```python
from build123d import *

# Parameters (mm, degrees)
SKETCH_1_W                         = 50
SKETCH_1_H                         = 140
SM_BASE_FLANGE_1_DEPTH             = 3
SM_EDGE_FLANGE_1_STRIP_W           = 13.4732
SM_EDGE_FLANGE_1_STRIP_H           = 3
SM_EDGE_FLANGE_1_STRIP_CUT_DEPTH   = 50
SM_EDGE_FLANGE_1_STRIP_2_W         = 13.4732
SM_EDGE_FLANGE_1_STRIP_2_H         = 3
SM_EDGE_FLANGE_1_STRIP_CUT_2_DEPTH = 50
SM_EDGE_FLANGE_1_DEPTH             = 50
SM_EDGE_FLANGE_1_BEND_DEPTH        = 50
SM_EDGE_FLANGE_2_STRIP_W           = 13.4732
SM_EDGE_FLANGE_2_STRIP_H           = 3
SM_EDGE_FLANGE_2_STRIP_CUT_DEPTH   = 50
SM_EDGE_FLANGE_2_STRIP_2_W         = 13.4732
SM_EDGE_FLANGE_2_STRIP_2_H         = 3
SM_EDGE_FLANGE_2_STRIP_CUT_2_DEPTH = 50
SM_EDGE_FLANGE_2_DEPTH             = 50
SM_EDGE_FLANGE_2_BEND_DEPTH        = 50
SKETCH_18_R                        = 6.5
CUT_EXTRUDE_1_DEPTH                = 179.686876966


# Sheet-metal steps are written as plain solids
with BuildPart() as part:
    # Sketch 1 → 基体-法兰1 (new body)
    with BuildSketch(Plane.XY):
        with Locations((25, 70)):
            Rectangle(SKETCH_1_W, SKETCH_1_H)
    extrude(amount=-SM_BASE_FLANGE_1_DEPTH)

    # 边线-法兰1 strip (across the edge) → 边线-法兰1 strip cut (cut)
    with BuildSketch(Plane(origin=(0, 140, -3), x_dir=(0, -1, 0), z_dir=(1, 0, 0))):
        with Locations((-6, -1.5)):
            Rectangle(SM_EDGE_FLANGE_1_STRIP_W, SM_EDGE_FLANGE_1_STRIP_H)
    extrude(amount=SM_EDGE_FLANGE_1_STRIP_CUT_DEPTH, mode=Mode.SUBTRACT)

    # 边线-法兰1 strip 2 (across the edge) → 边线-法兰1 strip cut 2 (cut)
    with BuildSketch(Plane(origin=(50, 0, -3), x_dir=(0, 1, 0), z_dir=(-1, 0, 0))):
        with Locations((-6, -1.5)):
            Rectangle(SM_EDGE_FLANGE_1_STRIP_2_W, SM_EDGE_FLANGE_1_STRIP_2_H)
    extrude(amount=SM_EDGE_FLANGE_1_STRIP_CUT_2_DEPTH, mode=Mode.SUBTRACT)

    # 边线-法兰1 section (across the edge) → 边线-法兰1 (add)
    with BuildSketch(Plane(origin=(0, 140, -3), x_dir=(0, -1, 0), z_dir=(1, 0, 0))):
        with BuildLine():
            Line((-3, 0.7366), (-3, 17))
            Line((-3, 17), (0, 17))
            Line((0, 17), (0, 0.7366))
            ThreePointArc((0, 0.7366), (0.215745145, 0.215745145), (0.7366, 0))
            Line((0.7366, 0), (0.7366, -3))
            ThreePointArc((0.7366, -3), (-1.905575199, -1.905575199), (-3, 0.7366))
        make_face()
    extrude(amount=SM_EDGE_FLANGE_1_DEPTH)

    # 边线-法兰1 section 2 (across the edge) → 边线-法兰1 bend (add)
    with BuildSketch(Plane(origin=(50, 0, -3), x_dir=(0, 1, 0), z_dir=(-1, 0, 0))):
        with BuildLine():
            Line((-3, 0.7366), (-3, 17))
            Line((-3, 17), (0, 17))
            Line((0, 17), (0, 0.7366))
            ThreePointArc((0, 0.7366), (0.215745145, 0.215745145), (0.7366, 0))
            Line((0.7366, 0), (0.7366, -3))
            ThreePointArc((0.7366, -3), (-1.905575199, -1.905575199), (-3, 0.7366))
        make_face()
    extrude(amount=SM_EDGE_FLANGE_1_BEND_DEPTH)

    # 边线-法兰2 strip (across the edge) → 边线-法兰2 strip cut (cut)
    with BuildSketch(Plane(origin=(0, -3, -20), x_dir=(0, 0, 1), z_dir=(1, 0, 0))):
        with Locations((-6, -1.5)):
            Rectangle(SM_EDGE_FLANGE_2_STRIP_W, SM_EDGE_FLANGE_2_STRIP_H)
    extrude(amount=SM_EDGE_FLANGE_2_STRIP_CUT_DEPTH, mode=Mode.SUBTRACT)

    # 边线-法兰2 strip 2 (across the edge) → 边线-法兰2 strip cut 2 (cut)
    with BuildSketch(Plane(origin=(50, 143, -20), x_dir=(0, 0, 1), z_dir=(-1, 0, 0))):
        with Locations((-6, -1.5)):
            Rectangle(SM_EDGE_FLANGE_2_STRIP_2_W, SM_EDGE_FLANGE_2_STRIP_2_H)
    extrude(amount=SM_EDGE_FLANGE_2_STRIP_CUT_2_DEPTH, mode=Mode.SUBTRACT)

    # 边线-法兰2 section (across the edge) → 边线-法兰2 (add)
    with BuildSketch(Plane(origin=(0, -3, -20), x_dir=(0, 0, 1), z_dir=(1, 0, 0))):
        with BuildLine():
            Line((-3, 0.7366), (-3, 27))
            Line((-3, 27), (0, 27))
            Line((0, 27), (0, 0.7366))
            ThreePointArc((0, 0.7366), (0.215745145, 0.215745145), (0.7366, 0))
            Line((0.7366, 0), (0.7366, -3))
            ThreePointArc((0.7366, -3), (-1.905575199, -1.905575199), (-3, 0.7366))
        make_face()
    extrude(amount=SM_EDGE_FLANGE_2_DEPTH)

    # 边线-法兰2 section 2 (across the edge) → 边线-法兰2 bend (add)
    with BuildSketch(Plane(origin=(50, 143, -20), x_dir=(0, 0, 1), z_dir=(-1, 0, 0))):
        with BuildLine():
            Line((-3, 0.7366), (-3, 27))
            Line((-3, 27), (0, 27))
            Line((0, 27), (0, 0.7366))
            ThreePointArc((0, 0.7366), (0.215745145, 0.215745145), (0.7366, 0))
            Line((0.7366, 0), (0.7366, -3))
            ThreePointArc((0.7366, -3), (-1.905575199, -1.905575199), (-3, 0.7366))
        make_face()
    extrude(amount=SM_EDGE_FLANGE_2_BEND_DEPTH)

    # 草图18 → 切除-拉伸1 (cut, through all)
    with BuildSketch(Plane.XY):
        with Locations((25, 70)):
            Circle(SKETCH_18_R)
    extrude(amount=-CUT_EXTRUDE_1_DEPTH, mode=Mode.SUBTRACT)


solid = part.part
```
Check sheet for the modelled part. Datum: model origin and axes. Units: mm. A direction names the side the tool comes from. Round coordinates to 2 decimals unless told otherwise and drop trailing zeros. Write each loop counter-clockwise with the first axis right and the second up, starting at its lowest first coordinate (ties: lowest second). Pieces come first, ordered by that corner, then holes. Notation, with made-up numbers: (-21.5, 42.25) -> (-16.5, 42.25) arc R23 ccw to (-16.5, 55.25) -> close; hole circle Ø8 at (-22.75, 6). An arc over 180 degrees is marked (long way). One line per question, with ' | ' between items. Start each with the question number.
1. Sectioned sample at D-D, the plane x = 44.5. Record the cut outline in (y, z), then the cut area to 3 significant figures.
2. Sectioned sample at C-C, the plane x = 25. Record the cut outline in (y, z), then the cut area to 3 significant figures.
3. Set-up check for faces 4 (the face through (14, 71, -3)), 5 (the face through (25, -3, -11)), 6 (the face through (25, 157, -20)): record each of +Z, -Z, +X, -X, +Y, -Y from which the full face is reachable in a straight line by a thin tool's end or side.
4. Release check for a two-part mould opening along Y. For faces 1 (the face through (50, 70, -2)), 2 (the face through (25, 143, -11)), 3 (the face through (25, 0, -12)) record: +Y half, -Y half, draft (parallel to the pull), parting line (faces both ways), or undercut.
5. Sectioned sample at B-B, the plane z = -16.5. Record the cut outline in (x, y).
6. Sectioned sample at A-A, the plane y = 70. Record the cut outline in (x, z), then the cut area to 3 significant figures.
7. Scan lines: line 1 along Y through (x, z) = (46.5, -16.5); line 2 along Z through (x, y) = (12.5, 146); line 3 along Y through (x, z) = (25, -2.25). Record each from-to range of solid material in increasing order. Write a range as from..to.
8. Depth check by flat-ended pin: pin 1 (3 mm diameter, centred on x = 6.5, z = -9, fed in from +Y); pin 2 (4 mm diameter, centred on x = 22.5, z = -13.5, fed in from -Y); pin 3 (21 mm diameter, centred on x = 31.5, y = 155, fed in from +Z). Enter the tip coordinate at first touch or a pass-through.
Taken from the geometry:
1) outline: (-30, -23) -> (-3.74, -23) arc R3.74 ccw to (0, -19.26) -> (0, -3.74) arc R0.74 cw to (0.74, -3) -> (139.26, -3) arc R0.74 cw to (140, -3.74) -> (140, -19.26) arc R3.74 ccw to (143.74, -23) -> (170, -23) -> (170, -20) -> (143.74, -20) arc R0.74 cw to (143, -19.26) -> (143, -3.74) arc R3.74 ccw to (139.26, 0) -> (0.74, 0) arc R3.74 ccw to (-3, -3.74) -> (-3, -19.26) arc R0.74 cw to (-3.74, -20) -> (-30, -20) -> close | area: 708 mm^2
2) outline: (-30, -23) -> (-3.74, -23) arc R3.74 ccw to (0, -19.26) -> (0, -3.74) arc R0.74 cw to (0.74, -3) -> (63.5, -3) -> (63.5, 0) -> (0.74, 0) arc R3.74 ccw to (-3, -3.74) -> (-3, -19.26) arc R0.74 cw to (-3.74, -20) -> (-30, -20) -> close; (76.5, -3) -> (139.26, -3) arc R0.74 cw to (140, -3.74) -> (140, -19.26) arc R3.74 ccw to (143.74, -23) -> (170, -23) -> (170, -20) -> (143.74, -20) arc R0.74 cw to (143, -19.26) -> (143, -3.74) arc R3.74 ccw to (139.26, 0) -> (76.5, 0) -> close | area: 669 mm^2
3) face 4: -Z, +X, -X | face 5: +Z, +X, -X, -Y | face 6: +Z, +X, -X, +Y
4) face 1: draft | face 2: +Y half | face 3: undercut
5) outline: (0, -3) -> (50, -3) -> (50, 0) -> (0, 0) -> close; (0, 140) -> (50, 140) -> (50, 143) -> (0, 143) -> close
6) outline: (0, -3) -> (18.5, -3) -> (18.5, 0) -> (0, 0) -> close; (31.5, -3) -> (50, -3) -> (50, 0) -> (31.5, 0) -> close | area: 111 mm^2
7) line 1: y = -3..0, 140..143 | line 2: z = -23..-20 | line 3: y = -2.69..63.5, 76.5..142.69
8) pin 1: stops at y = 143 | pin 2: stops at y = -3 | pin 3: stops at z = -20
